Here's how the part is built. I have some questions about the finished solid (model axes, mm). Round coordinates to 2 decimals unless told otherwise and drop trailing zeros. Order: outer loops, then holes, each group sorted by start corner. A loop starts at its lowest first (then second) coordinate and runs counter-clockwise, first axis right, second up.
Autodesk Inventor part; units mm, degrees
ref_plane "YZ Plane" through (0, 0, 0) normal (1, 0, 0) x (0, 1, 0)
ref_plane "XZ Plane" through (0, 0, 0) normal (0, 1, 0) x (-1, 0, 0)
ref_plane "XY Plane" through (0, 0, 0) normal (0, 0, 1) x (1, 0, 0)
sketch "Sketch3" plane through (0, 0, 0) normal (0, 1, 0) x (-1, 0, 0)
  line L0 (0.77, 1.27) -> (-0.77, 1.27)
  line L1 (-1.27, 0.77) -> (-1.27, -0.77)
  line L2 (-0.77, -1.27) -> (0.77, -1.27)
  line L3 (1.27, -0.77) -> (1.27, 0.77)
  line L4 (1.27, 0.77) -> (0.77, 1.27)
  line L5 (-0.77, 1.27) -> (-1.27, 0.77)
  line L6 (-1.27, -0.77) -> (-0.77, -1.27)
  line L7 (0.77, -1.27) -> (1.27, -0.77)
  point P0 (0, 0)
  point P1 (-1.27, 0)
  point P2 (0, -1.27)
  dimension "d6" = 2.54
  dimension "d7" = 0.5
  dimension "d8" = 45
extrude "Extrusion3" add sketch "Sketch3" along normal blind 2.54
sketch "Sketch4" plane through (0, 2.54, 0) normal (0, 1, 0) x (1, 0, 0)
  line L0 (-0.25, -0.25) -> (0.25, -0.25)
  line L1 (0.25, -0.25) -> (0.25, 0.25)
  line L2 (0.25, 0.25) -> (-0.25, 0.25)
  line L3 (-0.25, 0.25) -> (-0.25, -0.25)
  point P0 (0, 0)
  point P1 (0, 0.25)
  point P2 (-0.25, 0)
  dimension "d11" = 0.5
extrude "Extrusion4" add sketch "Sketch4" along normal blind 6.5
sketch "Sketch5" plane through (0, 0, 0) normal (0, -1, 0) x (1, 0, 0)
  circle A0 centre (0, 0) radius 0.25
  dimension "d14" = 0.5
extrude "Extrusion5" add sketch "Sketch5" along normal blind 3
properties part number "Pin-round-2.54-male"
1. If we section it at B-B, the plane x = 0: Write out the boundary of the cut face in (y, z).
Evaluation:
outline: (-3, -0.25) - (0, -0.25) - (0, -1.27) - (2.54, -1.27) - (2.54, -0.25) - (9.04, -0.25) - (9.04, 0.25) - (2.54, 0.25) - (2.54, 1.27) - (0, 1.27) - (0, 0.25) - (-3, 0.25) - close
2. If we section it at C-C, the plane y = 0.5: Write out the boundary of the cut face in (x, z), and give its area (3 significant figures).
Evaluation:
outline: (-1.27, -0.77) - (-0.77, -1.27) - (0.77, -1.27) - (1.27, -0.77) - (1.27, 0.77) - (0.77, 1.27) - (-0.77, 1.27) - (-1.27, 0.77) - close
area: 5.95 mm2
3. If we section it at A-A, the plane z = 0: Write out the boundary of the cut face in (x, y).
Evaluation:
outline: (-1.27, 0) - (-0.25, 0) - (-0.25, -3) - (0.25, -3) - (0.25, 0) - (1.27, 0) - (1.27, 2.54) - (0.25, 2.54) - (0.25, 9.04) - (-0.25, 9.04) - (-0.25, 2.54) - (-1.27, 2.54) - close
4. If we section it at D-D, the plane y = -1.5: Write out the boundary of the cut face in (x, z), and give its area (3 significant figures).
Evaluation:
outline: circle Ø0.5 at (0, 0)
area: 0.196 mm2
5. I'm going to push flat-ended pins straight in: P1, Ø0.6, axis at x = 0, y = 5, coming from the -Z side; P2, Ø1.3, axis at x = -0.5, z = 0, coming from the +Y side; P3, Ø0.6, axis at y = 5.5, z = 0, coming from the -X side; P4, Ø1.5, axis at x = 1, z = -0.5, coming from the +Y side. Where does each tip first touch, or does it pass through?
Evaluation:
P1: stops at z = -0.25
P2: stops at y = 9.04
P3: stops at x = -0.25
P4: stops at y = 2.54
6. I need wall thicknesses on probe 1 along Y at (x, z) = (0.4, -0.6); probe 2 along Z at (x, y) = (0.2, 8.25). Which ranges of each line are inside material? Lowest first, please.
Evaluation:
probe 1: y = 0 to 2.54
probe 2: z = -0.25 to 0.25
7. If we mould it in two halves opening along Y, with no side actions, what happens to faces 1 (the flat face through (-0.3, 0, 0.3)), 2 (the flat face through (1.27, 1, 0))? For each: released by +Y, released by -Y, zero draft, split by the parting line, or undercut.
Evaluation:
face 1: released by -Y
face 2: zero draft
